Read the model definition and answer for the solid it produces. Units are mm, in the model's axes. Face numbers are marked on the shaded views. Coordinates: 2 decimals unless noted, no trailing zeros. Write each loop counter-clockwise with the first axis right and the second up, starting at its lowest first coordinate (ties: lowest second). Pieces come first, ordered by that corner, then holes. Notation, with made-up numbers: (-38, 0) -> (-8, 0) arc R6 ccw to (-8, 11) -> close; hole circle Ø2 at (-26, -28). An arc over 180 degrees is marked (long way). One line per item, written item: value. Start each with the question number.
1. Find section A-A, the plane z = 3. Write down the section's boundary in (x, y), and give its area (3 significant figures).
2. Find section C-C, the plane x = -16.5. Write down the section's boundary in (y, z), and give its area (3 significant figures).
3. Consider line 1 along Z through (x, y) = (4, 12.25); line 2 along Y through (x, z) = (-30.5, 0.8); line 3 along X through (y, z) = (11.5, 4). Determine where each line is inside the solid, lowest interval first.
4. Find section B-B, the plane y = 12.75. Write down the section's boundary in (x, z), and give its area (3 significant figures).
5. For a pull along X with two mould halves and no side action, classify the marked faces 1 and 2 as pulls with the +X half, pulls with the -X half, needs draft (parallel to the pull), parting line crosses it, or undercut.
6. Given P1, Ø1, axis at x = -30, z = 0.5, coming from the +Y side; P2, Ø1.5, axis at y = 9.5, z = 2.5, coming from the +X side; P3, Ø1, axis at x = -31.5, y = 8, coming from the +Z side; P4, Ø4, axis at x = -30, y = 12, coming from the -Z side, each flat-ended and moving along its own axis, determine where each tip first touches the part or whether it passes through.
```python
from build123d import *

# Parameters (mm, degrees)
F1_DEPTH = 2
F3_DEPTH = 5
F5_DEPTH = 5


with BuildPart() as f1:
    # F0 (on Top) → F1 (new body)
    with BuildSketch(Plane.XY):
        Polygon((47.731567, 14.58858), (-58.212683, 14.58858), (-64.16142, 10.906025), (-58.212683, 6.940198), (47.731567, 6.940198), (55.096671, 11.472573), align=None)
    extrude(amount=F1_DEPTH)

    # F2 (on Top) → F3 (join)
    with BuildSketch(Plane.XY):
        Polygon((-58.495954, 14.305307), (-63.878149, 10.906025), (-58.495954, 6.940198), align=None)
    extrude(amount=F3_DEPTH)

    # F4 (on Top) → F5 (join)
    with BuildSketch(Plane.XY):
        Polygon((55.096671, 11.472573), (47.731567, 14.871853), (47.731567, 7.506745), align=None)
    extrude(amount=F5_DEPTH)


solid = f1.part
```
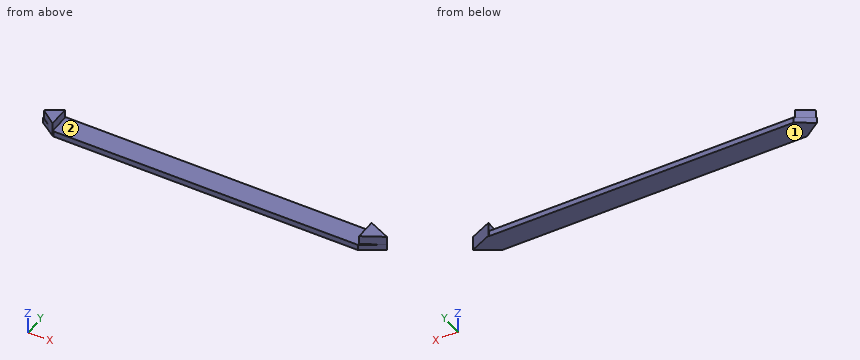
Answer block:
1. outline: (-63.88, 10.91) -> (-58.5, 6.94) -> (-58.5, 14.31) -> close; (47.73, 7.51) -> (55.1, 11.47) -> (47.73, 14.87) -> close
1. area: 46.9 mm2
2. outline: (6.94, 0) -> (14.59, 0) -> (14.59, 2) -> (6.94, 2) -> close
2. area: 15.3 mm2
3. line 1: z = 0 to 2
3. line 2: y = 6.94 to 14.59
3. line 3: x = -62.94 to -58.5, 47.73 to 55.04
4. outline: (-61.18, 0) -> (52.33, 0) -> (52.33, 5) -> (47.73, 5) -> (47.73, 2) -> (-58.5, 2) -> (-58.5, 5) -> (-60.96, 5) -> (-60.96, 2) -> (-61.18, 2) -> close
4. area: 248 mm2
5. face 1: needs draft
5. face 2: undercut
6. P1: stops at y = 14.59
6. P2: stops at x = 52.83
6. P3: stops at z = 2
6. P4: stops at z = 0
